```python
from build123d import *

# Parameters (mm, degrees)
BOSS_EXTRUDE1_DEPTH     = 3.175
CUT_EXTRUDE1_DEPTH      = 178.828345955
CAVITY1_START           = 31.75
CAVITY1_OUTLINE_W       = 6.35
CAVITY1_OUTLINE_H       = 6.35
CAVITY1_DEPTH           = 50.8
FILLET1_R               = 6.35
CUT_EXTRUDE2_DEPTH      = 178.828345955
FILLET2_R               = 6.35
F_1_4_CLEARANCE_HOLE1_D = 6.7564


# Read off the part's stored shape, not the designer's step: Cavity1
with BuildPart() as part:
    # Sketch1 → Boss-Extrude1 (new, symmetric)
    with BuildSketch(Plane.XY):
        Polygon((133.35, -3.175), (133.35, 117.475), (107.95, 117.475), (0, 9.525), (-107.95, 117.475), (-133.35, 117.475), (-133.35, -3.175), (-82.55, -3.175), (-82.55, -9.525), (-25.4, -9.525), (-25.4, -3.175), (25.4, -3.175), (25.4, -9.525), (82.55, -9.525), (82.55, -3.175), align=None)
    extrude(amount=BOSS_EXTRUDE1_DEPTH, both=True)

    # Sketch2 → Cut-Extrude1 (cut, through all)
    with BuildSketch(Plane.XY.offset(3.175)):
        Polygon((-8.980256121, 18.505256121), (-13.470384182, 14.015128061), (-31.430896424, 31.975640303), (-26.940768363, 36.465768363), align=None)
        Polygon((-62.861792847, 72.386792847), (-67.351920908, 67.896664787), (-49.391408666, 49.936152545), (-44.901280605, 54.426280605), align=None)
        Polygon((-98.782817332, 108.307817332), (-103.272945392, 103.817689271), (-85.31243315, 85.857177029), (-80.82230509, 90.34730509), align=None)
        Polygon((80.82230509, 90.34730509), (98.782817332, 108.307817332), (103.272945392, 103.817689271), (85.31243315, 85.857177029), align=None)
        Polygon((44.901280605, 54.426280605), (62.861792847, 72.386792847), (67.351920908, 67.896664787), (49.391408666, 49.936152545), align=None)
        Polygon((26.940768363, 36.465768363), (31.430896424, 31.975640303), (13.470384182, 14.015128061), (8.980256121, 18.505256121), align=None)
    extrude(amount=-CUT_EXTRUDE1_DEPTH, mode=Mode.SUBTRACT)

    # Cavity1 outline → Cavity1 (cut)
    with BuildSketch(Plane(origin=(0, 0, 0), x_dir=(1, 0, 0), z_dir=(0, 1, 0)).offset(CAVITY1_START)):
        with Locations((130.175, 0)):
            Rectangle(CAVITY1_OUTLINE_W, CAVITY1_OUTLINE_H)
        with Locations((-130.175, 0)):
            Rectangle(CAVITY1_OUTLINE_W, CAVITY1_OUTLINE_H)
    extrude(amount=CAVITY1_DEPTH, mode=Mode.SUBTRACT)

    # Fillet1
    fillet1_edges = [part.edges().sort_by_distance(p)[0] for p in [
        (0, 9.525, 0),
    ]]
    fillet(fillet1_edges, radius=FILLET1_R)

    # Sketch3 → Cut-Extrude2 (cut, through all)
    with BuildSketch(Plane.XY.offset(3.175)):
        Polygon((-101.6, 66.223719395), (-57.601280605, 22.225), (-101.6, 22.225), (-101.6, 31.75), align=None)
    cut_extrude2 = extrude(amount=-CUT_EXTRUDE2_DEPTH, mode=Mode.SUBTRACT)

    # Mirror1: Cut-Extrude2 across plane
    add(cut_extrude2.mirror(Plane(origin=(0, 0, 0), x_dir=(0, 0, 1), z_dir=(1, 0, 0))), mode=Mode.SUBTRACT)

    # Fillet2
    fillet2_edges = [part.edges().sort_by_distance(p)[0] for p in [
        (-57.601280605, 22.225, 0),
        (-101.6, 22.225, 0),
        (-101.6, 66.223719395, 0),
        (101.6, 22.225, 0),
        (57.601280605, 22.225, 0),
        (101.6, 66.223719395, 0),
    ]]
    fillet(fillet2_edges, radius=FILLET2_R)

    # 1/4 Clearance Hole1 (through all)
    with Locations(Plane.XY.offset(3.175)):
        with Locations((-47.473930622, 18.030114286)):
            f_1_4_clearance_hole1 = Hole(F_1_4_CLEARANCE_HOLE1_D / 2)

    # Mirror2: 1/4 Clearance Hole1 across plane
    add(f_1_4_clearance_hole1.mirror(Plane(origin=(0, 0, 0), x_dir=(0, 0, 1), z_dir=(1, 0, 0))), mode=Mode.SUBTRACT)


solid = part.part
```
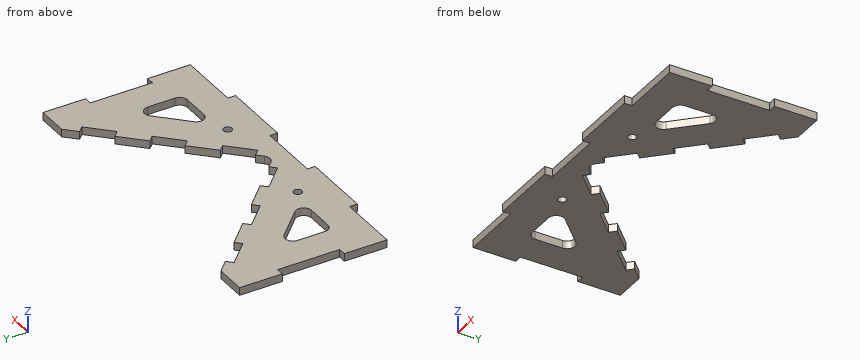
Part model, mm, in its own coordinate system. Give positions to 0.01 mm unless a question says otherwise; leave off trailing zeros. Order: outer loops, then holes, each group sorted by start corner. A loop starts at its lowest first (then second) coordinate and runs counter-clockwise, first axis right, second up. Notation, with made-up numbers: M 24,-4 L 48,-4 A15 cw 48,22 Z; hole C 53.5,30 d3. An arc over 180 degrees is marked long. Use a Markdown table: item, result. Add a question column.
(1) Drop flat-ended pins along their axis: P1, Ø1.9, axis at y = 66.5, z = 1.5, coming from the +X side; P2, Ø1, axis at x = 83.5, z = -2.5, coming from the -Y side (3 decimals); P3, Ø1.9, axis at y = -7, z = 1, coming from the -X side; P4, Ø6, axis at x = 47.47, y = 18.03, coming from the +Z side. Give the stop position or say it passes through.
(2) Saw through at C-C, the plane x = -16. Give the cut face in (y, z) (3 decimals).
(3) Probe line 1 along X through (y, z) = (53, -0.5) (3 decimals); line 2 along X through (y, z) = (45, 3) (3 decimals); line 3 along X through (y, z) = (20, 2.25). List the from-to ranges inside material, lowest first. Write a range as [from, to].
(4) Saw through at A-A, the plane y = 64. Give the cut face in (x, z) (3 decimals), and give its area (3 significant figures).
(5) Saw through at B-B, the plane z = 0. Give the number of separate pieces and of enclosed holes in the cut face, and give its area (3 significant figures).
Answer key:
| question | item | result |
|---|---|---|
| 1 | P1 | x = 127 |
| 1 | P2 | y = -3.175 |
| 1 | P3 | x = -82.55 |
| 1 | P4 | through |
| 2 | outline | M -3.175,-3.175 L 16.545,-3.175 L 16.545,3.175 L -3.175,3.175 Z |
| 3 | line 1 | [-127, -101.24], [-88.376, -52.455], [-46.328, -43.475], [43.475, 46.328], [52.455, 88.376], [101.24, 127] |
| 3 | line 2 | [-127, -101.6], [-80.376, -35.475], [35.475, 80.376], [101.6, 127] |
| 3 | line 3 | [-133.35, -50.22], [-44.73, -19.46], [19.46, 44.73], [50.22, 133.35] |
| 4 | outline | M -127,-3.175 L -63.455,-3.175 L -63.455,3.175 L -127,3.175 Z; M 63.455,-3.175 L 127,-3.175 L 127,3.175 L 63.455,3.175 Z |
| 4 | area | 807 mm^2 |
| 5 | separate pieces | 1 |
| 5 | enclosed holes | 4 |
| 5 | area | 17,900 mm^2 |
